Model file for the job. Use its own axes, mm. Round coordinates to 2 decimals unless told otherwise and drop trailing zeros. Put each result on its own line as item: value. Start each with the question number.
Q1. Flat gauge pins, fed straight in: P1, Ø1.3, axis at y = 3.5, z = 331, coming from the +X side; P2, Ø1, axis at x = 3, z = 69, coming from the +Y side; P3, Ø1.3, axis at x = 1.5, z = 370, coming from the +Y side. Where does each tip first touch, or does it go through?
Q2. Probe L1, parallel to Y at x = 0, z = 337.5; L2, parallel to X at y = -0.75, z = 439; L3, parallel to Y at x = -5, z = 94. List the from-to ranges inside material, lowest first.
Q3. Cut at A-A, the plane z = 366. State how many separate pieces and enclosed holes the cut face has, and give its area (3 significant figures).
from build123d import *

# Parameters (mm, degrees)
F0_R     = 2.1
F1_DEPTH = 545


with BuildPart() as f1:
    # F0 (on Top) → F1 (new body)
    with BuildSketch(Plane.XY):
        with BuildLine():
            Line((10, 4.410115), (10, 8.270115))
            ThreePointArc((10, 8.270115), (9.56066, 9.330775), (8.5, 9.770115))
            Line((8.5, 9.770115), (4.64, 9.770115))
            Line((4.64, 9.770115), (2.84, 7.970115))
            Line((2.84, 7.970115), (5.49934, 7.970115))
            Line((5.49934, 7.970115), (5.49934, 6.330115))
            Line((5.49934, 6.330115), (2.84, 3.670775))
            Line((2.84, 3.670775), (0.25, 3.670775))
            Line((0.25, 3.670775), (0, 3.420775))
            Line((0, 3.420775), (-0.25, 3.670775))
            Line((-0.25, 3.670775), (-2.84, 3.670775))
            Line((-2.84, 3.670775), (-5.49934, 6.330115))
            Line((-5.49934, 6.330115), (-5.49934, 7.970115))
            Line((-5.49934, 7.970115), (-2.84, 7.970115))
            Line((-2.84, 7.970115), (-4.64, 9.770115))
            Line((-4.64, 9.770115), (-8.5, 9.770115))
            ThreePointArc((-8.5, 9.770115), (-9.56066, 9.330775), (-10, 8.270115))
            Line((-10, 8.270115), (-10, 4.410115))
            Line((-10, 4.410115), (-8.2, 2.610115))
            Line((-8.2, 2.610115), (-8.2, 5.269455))
            Line((-8.2, 5.269455), (-6.56, 5.269455))
            Line((-6.56, 5.269455), (-3.90066, 2.610115))
            Line((-3.90066, 2.610115), (-3.90066, 0.020115))
            Line((-3.90066, 0.020115), (-3.65066, -0.229885))
            Line((-3.65066, -0.229885), (-3.90066, -0.479885))
            Line((-3.90066, -0.479885), (-3.90066, -3.069885))
            Line((-3.90066, -3.069885), (-6.56, -5.729225))
            Line((-6.56, -5.729225), (-8.2, -5.729225))
            Line((-8.2, -5.729225), (-8.2, -3.069885))
            Line((-8.2, -3.069885), (-10, -4.869885))
            Line((-10, -4.869885), (-10, -8.729885))
            ThreePointArc((-10, -8.729885), (-9.56066, -9.790545), (-8.5, -10.229885))
            Line((-8.5, -10.229885), (-4.64, -10.229885))
            Line((-4.64, -10.229885), (-2.84, -8.429885))
            Line((-2.84, -8.429885), (-5.49934, -8.429885))
            Line((-5.49934, -8.429885), (-5.49934, -6.789885))
            Line((-5.49934, -6.789885), (-2.84, -4.130545))
            Line((-2.84, -4.130545), (-0.25, -4.130545))
            Line((-0.25, -4.130545), (0, -3.880545))
            Line((0, -3.880545), (0.25, -4.130545))
            Line((0.25, -4.130545), (2.84, -4.130545))
            Line((2.84, -4.130545), (5.49934, -6.789885))
            Line((5.49934, -6.789885), (5.49934, -8.429885))
            Line((5.49934, -8.429885), (2.84, -8.429885))
            Line((2.84, -8.429885), (4.64, -10.229885))
            Line((4.64, -10.229885), (8.5, -10.229885))
            ThreePointArc((8.5, -10.229885), (9.56066, -9.790545), (10, -8.729885))
            Line((10, -8.729885), (10, -4.869885))
            Line((10, -4.869885), (8.2, -3.069885))
            Line((8.2, -3.069885), (8.2, -5.729225))
            Line((8.2, -5.729225), (6.56, -5.729225))
            Line((6.56, -5.729225), (3.90066, -3.069885))
            Line((3.90066, -3.069885), (3.90066, -0.479885))
            Line((3.90066, -0.479885), (3.65066, -0.229885))
            Line((3.65066, -0.229885), (3.90066, 0.020115))
            Line((3.90066, 0.020115), (3.90066, 2.610115))
            Line((3.90066, 2.610115), (6.56, 5.269455))
            Line((6.56, 5.269455), (8.2, 5.269455))
            Line((8.2, 5.269455), (8.2, 2.610115))
            Line((8.2, 2.610115), (10, 4.410115))
        make_face()
        Polygon((-6.56934, -7.859885), (-6.56934, -8.429885), (-8.2, -8.429885), (-8.2, -6.799225), (-7.63, -6.799225), align=None, mode=Mode.SUBTRACT)
        Polygon((8.2, -8.429885), (6.56934, -8.429885), (6.56934, -7.859885), (7.63, -6.799225), (8.2, -6.799225), align=None, mode=Mode.SUBTRACT)
        Polygon((-7.63, 6.339455), (-8.2, 6.339455), (-8.2, 7.970115), (-6.56934, 7.970115), (-6.56934, 7.400115), align=None, mode=Mode.SUBTRACT)
        with Locations((0, -0.229885)):
            Circle(F0_R, mode=Mode.SUBTRACT)
        Polygon((6.56934, 7.400115), (6.56934, 7.970115), (8.2, 7.970115), (8.2, 6.339455), (7.63, 6.339455), align=None, mode=Mode.SUBTRACT)
    extrude(amount=F1_DEPTH)


solid = f1.part
Ans:
1. P1: stops at x = 9.74
1. P2: stops at y = 8.63
1. P3: stops at y = 3.67
2. L1: y = -3.88 to -2.33, 1.87 to 3.42
2. L2: x = -3.9 to -2.03, 2.03 to 3.9
2. L3: y = -10.23 to -8.43, -6.29 to -4.17, 3.71 to 5.83, 7.97 to 9.77
3. separate pieces: 1
3. enclosed holes: 5
3. area: 161 mm^2
